```python
from build123d import *

# Parameters (mm, degrees)
SKETCH1_R           = 11
BOSS_EXTRUDE1_DEPTH = 3
SKETCH2_R           = 1.5
CUT_EXTRUDE1_DEPTH  = 5
SKETCH3_R           = 5
BOSS_EXTRUDE2_DEPTH = 10
SKETCH4_R           = 4
CUT_EXTRUDE2_DEPTH  = 21.273134933


with BuildPart() as part:
    # Sketch1 → Boss-Extrude1 (new body)
    with BuildSketch(Plane(origin=(0, 0, 0), x_dir=(1, 0, 0), z_dir=(0, 1, 0))):
        with Locations(Location((0, 0, 0), (0, 0, 270))):
            Circle(SKETCH1_R)
    extrude(amount=BOSS_EXTRUDE1_DEPTH)

    # Sketch2 → Cut-Extrude1 (cut)
    with BuildSketch(Plane(origin=(0, 3, 0), x_dir=(1, 0, 0), z_dir=(0, 1, 0))):
        with Locations(Location((-5.617707867, 5.617707867, 0), (0, 0, 270))):
            Circle(SKETCH2_R)
        with Locations(Location((5.617707867, 5.617707867, 0), (0, 0, 270))):
            Circle(SKETCH2_R)
        with Locations(Location((-5.617707867, -5.617707867, 0), (0, 0, 270))):
            Circle(SKETCH2_R)
        with Locations(Location((5.617707867, -5.617707867, 0), (0, 0, 270))):
            Circle(SKETCH2_R)
    extrude(amount=-CUT_EXTRUDE1_DEPTH, mode=Mode.SUBTRACT)

    # Sketch3 → Boss-Extrude2 (add)
    with BuildSketch(Plane(origin=(0, 3, 0), x_dir=(1, 0, 0), z_dir=(0, 1, 0))):
        with Locations(Location((0, 0, 0), (0, 0, 270))):
            Circle(SKETCH3_R)
    extrude(amount=BOSS_EXTRUDE2_DEPTH)

    # Sketch4 → Cut-Extrude2 (cut, through all)
    with BuildSketch(Plane(origin=(0, 13, 0), x_dir=(1, 0, 0), z_dir=(0, 1, 0))):
        with Locations(Location((0, 0, 0), (0, 0, 270))):
            Circle(SKETCH4_R)
    extrude(amount=-CUT_EXTRUDE2_DEPTH, mode=Mode.SUBTRACT)


solid = part.part
```
The model under review builds one solid part; all positions refer to its coordinate system, in mm. A direction names the side the tool comes from. Give positions to 0.01 mm unless a question says otherwise; leave off trailing zeros. Write each loop counter-clockwise with the first axis right and the second up, starting at its lowest first coordinate (ties: lowest second). Pieces come first, ordered by that corner, then holes. Notation, with made-up numbers: (67, -39.75) - (86, -39.75) arc R14 cw to (86, -35.75) - close; hole circle Ø7 at (42.5, 84). An arc over 180 degrees is marked (long way). Answer in a Markdown table with one row per item. Add a question column.
1. Wall thickness on line 1 along X through (y, z) = (2, 6.75); line 2 along Z through (x, y) = (-5, 1.5); line 3 along Y through (x, z) = (-3, -9.5): over which ranges is each line inside the solid? List them lowest first. Write a range as [from, to].
2. Tool access review of faces 5 (the cylindrical face through (-6.95, 1.52, 6.31)), 6 (the flat face through (-2, 3, 5)): name each direction out of +Z, -Z, +X, -X, +Y, -Y from which nothing blocks a thin tool from reaching the whole face with its end or side.
3. We need section B-B on x = 0. Write out the cut boundary in (y, z).
4. Insertion check: P1, Ø3, axis at x = 6.5, y = 2.5, coming from the -Z side; P2, Ø1.5, axis at y = 8.5, z = -4, coming from the +X side; P3, Ø1, axis at x = 7, z = 8, coming from the +Y side. Each pin has a flat end and moves straight along its axis. Give the tip position at first contact, or say it passes through.
5. Draft analysis for pull direction Z (two halves, no side actions). For faces 1 (the cylindrical face through (-4.88, 7.93, -1.08)), 2 (the flat face through (-5, 0, 0)), 3 (the cylindrical face through (6.883, 1.521, 6.424)), 4 (the cylindrical face through (-7.082, 1.521, -5.943)), state which applies: +Z half, -Z half, draft (parallel to the pull), parting line (faces both ways), or undercut.
6. We need section A-A on z = 0. Write out the cut boundary in (x, y), then the cut area to 3 significant figures.
7. We need section C-C on y = 6. Write out the cut boundary in (x, z), then the cut area to 3 significant figures.
8. We need section D-D on z = -6. Write out the cut boundary in (x, y), then the cut area to 3 significant figures.
Ans:
| question | item | result |
|---|---|---|
| 1 | line 1 | x = [-8.69, -6.6], [-4.63, 4.63], [6.6, 8.69] |
| 1 | line 2 | z = [-9.8, -6.98], [-4.25, 4.25], [6.98, 9.8] |
| 1 | line 3 | y = [0, 3] |
| 2 | face 5 | +Y, -Y |
| 2 | face 6 | +Y |
| 3 | outline | (0, -11) - (3, -11) - (3, -5) - (13, -5) - (13, -4) - (0, -4) - close; (0, 4) - (13, 4) - (13, 5) - (3, 5) - (3, 11) - (0, 11) - close |
| 4 | P1 | stops at z = -9.8 |
| 4 | P2 | stops at x = 3.8 |
| 4 | P3 | stops at y = 3 |
| 5 | face 1 | parting line |
| 5 | face 2 | draft |
| 5 | face 3 | undercut |
| 5 | face 4 | undercut |
| 6 | outline | (-11, 0) - (-4, 0) - (-4, 13) - (-5, 13) - (-5, 3) - (-11, 3) - close; (4, 0) - (11, 0) - (11, 3) - (5, 3) - (5, 13) - (4, 13) - close |
| 6 | area | 62.0 mm^2 |
| 7 | outline | circle Ø10 at (0, 0); hole circle Ø8 at (0, 0) |
| 7 | area | 28.3 mm^2 |
| 8 | outline | (-9.22, 0) - (-7.07, 0) - (-7.07, 3) - (-9.22, 3) - close; (-4.17, 0) - (4.17, 0) - (4.17, 3) - (-4.17, 3) - close; (7.07, 0) - (9.22, 0) - (9.22, 3) - (7.07, 3) - close |
| 8 | area | 37.9 mm^2 |
